from build123d import *

# Parameters (mm, degrees)
CROQUIS1_W              = 120
CROQUIS1_H              = 75
SALIENTE_EXTRUIR1_DEPTH = 7
CROQUIS2_W              = 73
CROQUIS2_H              = 50
CORTAR_EXTRUIR1_DEPTH   = 15
CROQUIS3_W              = 88
CROQUIS3_H              = 56
CORTAR_EXTRUIR2_DEPTH   = 6
CROQUIS4_W              = 23.5
CROQUIS4_H              = 10.5
CORTAR_EXTRUIR3_DEPTH   = 25
CHAFL_N3_SIZE           = 7


with BuildPart() as part:
    # Croquis1 → Saliente-Extruir1 (new body)
    with BuildSketch(Plane.XY):
        Rectangle(CROQUIS1_W, CROQUIS1_H)
    extrude(amount=SALIENTE_EXTRUIR1_DEPTH)

    # Croquis2 → Cortar-Extruir1 (cut)
    with BuildSketch(Plane(origin=(0, 0, 0), x_dir=(-1, 0, 0), z_dir=(0, 0, -1))):
        Rectangle(CROQUIS2_W, CROQUIS2_H)
    extrude(amount=-CORTAR_EXTRUIR1_DEPTH, mode=Mode.SUBTRACT)

    # Croquis3 → Cortar-Extruir2 (cut)
    with BuildSketch(Plane.XY.offset(7)):
        Rectangle(CROQUIS3_W, CROQUIS3_H)
    extrude(amount=-CORTAR_EXTRUIR2_DEPTH, mode=Mode.SUBTRACT)

    # Croquis4 → Cortar-Extruir3 (cut)
    with BuildSketch(Plane(origin=(0, 0, 0), x_dir=(-1, 0, 0), z_dir=(0, 0, -1))):
        with Locations((48.25, 0)):
            Rectangle(CROQUIS4_W, CROQUIS4_H)
    extrude(amount=-CORTAR_EXTRUIR3_DEPTH, mode=Mode.SUBTRACT)

    # Chaflán3
    chafl_n3_edges = [part.edges().sort_by_distance(p)[0] for p in [
        (-60, 37.5, 3.5),
        (60, 37.5, 3.5),
        (60, -37.5, 3.5),
        (-60, -37.5, 3.5),
    ]]
    chamfer(chafl_n3_edges, length=CHAFL_N3_SIZE)


solid = part.part
Verification items for the finished model (mm, model axes). A direction names the side the tool comes from. Coordinates: 2 decimals unless noted, no trailing zeros. Loops run counter-clockwise (first coordinate to the right, second up) from the corner with the lowest first, then second, coordinate; pieces in that order, holes last. Notation, with made-up numbers: (32, -31.5) -> (49, -31.5) arc R22 cw to (49, -8.5) -> close; hole circle Ø10 at (-35.5, 55). An arc over 180 degrees is marked (long way). Write each question's results on one line, items separated by ' | '.
Item 1: Section check C-C, the plane z = 2.25. Enter the section's corners in (x, y).
Found:
outline: (-60, -30.5) -> (-53, -37.5) -> (53, -37.5) -> (60, -30.5) -> (60, 30.5) -> (53, 37.5) -> (-53, 37.5) -> (-60, 30.5) -> (-60, 5.25) -> (-44, 5.25) -> (-44, 28) -> (44, 28) -> (44, -28) -> (-44, -28) -> (-44, -5.25) -> (-60, -5.25) -> close
Item 2: Gauge pin test, flat ends, axial feed: pin 1 (0.5 mm diameter, centred on y = -2.5, z = 0.5, fed in from -X); pin 2 (12 mm diameter, centred on x = 27.5, y = 15, fed in from +Z). Record the tip position at first contact, or that the pin passes through.
Found:
pin 1: stops at x = 36.5 | pin 2: passes through
Item 3: Mould release check, pull along X, two halves, no side actions. Record for faces 4 (the face through (-60, 18, 3)), 5 (the face through (-1, 26, 0)), 6 (the face through (-1, -28, 4)): +X half, -X half, draft (parallel to the pull), parting line (faces both ways), or undercut.
Found:
face 4: -X half | face 5: draft | face 6: undercut
Item 4: Section check B-B, the plane y = -19.5. Enter the section's corners in (x, z), plus the area to 3 significant figures.
Found:
outline: (-60, 0) -> (-36.5, 0) -> (-36.5, 1) -> (-44, 1) -> (-44, 7) -> (-60, 7) -> close; (36.5, 0) -> (60, 0) -> (60, 7) -> (44, 7) -> (44, 1) -> (36.5, 1) -> close | area: 239 mm2
Item 5: Tool access check on faces 1 (the face through (-51, -5.25, 3)), 2 (the face through (60, 0, 3)), 3 (the face through (44, 0, 4)). Record the directions out of +Z, -Z, +X, -X, +Y, -Y that give a thin tool (end or side, any length) a straight path to the whole face; none if there is none.
Found:
face 1: +Z, -Z, -X | face 2: +Z, -Z, +X, +Y, -Y | face 3: +Z
Item 6: Section check A-A, the plane x = -14.5. Enter the section's corners in (y, z), plus the area to 3 significant figures.
Found:
outline: (-37.5, 0) -> (-25, 0) -> (-25, 1) -> (-28, 1) -> (-28, 7) -> (-37.5, 7) -> close; (25, 0) -> (37.5, 0) -> (37.5, 7) -> (28, 7) -> (28, 1) -> (25, 1) -> close | area: 139 mm2
Item 7: Section check D-D, the plane x = -51.5. Enter the section's corners in (y, z), plus the area to 4 significant figures.
Found:
outline: (-37.5, 0) -> (-5.25, 0) -> (-5.25, 7) -> (-37.5, 7) -> close; (5.25, 0) -> (37.5, 0) -> (37.5, 7) -> (5.25, 7) -> close | area: 451.5 mm2
Item 8: Material ranges on L1, parallel to Y at x = -29.5, z = 2; L2, parallel to X at y = 16, z = 4; L3, parallel to Y at x = -47, z = 2, recorded low to high.
Found:
L1: y = -37.5 to -28, 28 to 37.5 | L2: x = -60 to -44, 44 to 60 | L3: y = -37.5 to -5.25, 5.25 to 37.5
